Check sheet for the modelled part. Datum: model origin and axes. Units: mm. Coordinates: 2 decimals unless noted, no trailing zeros. Write each loop counter-clockwise with the first axis right and the second up, starting at its lowest first coordinate (ties: lowest second). Pieces come first, ordered by that corner, then holes. Notation, with made-up numbers: (54, -30.75) - (73, -30.75) arc R21 cw to (73, -8.75) - close; hole circle Ø8 at (71.25, 31.5). An arc over 180 degrees is marked (long way). Use one line per item in the form item = value. Start each with the question number.
1. Cross-section at A-A on z = -156.5. Record the boundary of the cut face in (x, y), then the cut area to 3 significant figures.
2. Go/stop test with flat-tipped pins: pin 1 Ø6 at (x, z) = (0, 195) entering from +Y; pin 2 Ø1.5 at (x, y) = (10, 1) entering from -Z; pin 3 Ø1.5 at (y, z) = (-1, -207) entering from +X. Record where each tip stops, or that it passes through.
3. Cross-section at B-B on y = 0.55. Record the boundary of the cut face in (x, z) (3 decimals).
4. Scan lines: line 1 along Z through (x, y) = (0, -0.4) (3 decimals); line 2 along X through (y, z) = (-1.35, 195) (3 decimals); line 3 along Z through (x, y) = (-4.5, -2). Record each from-to range of solid material in increasing order.
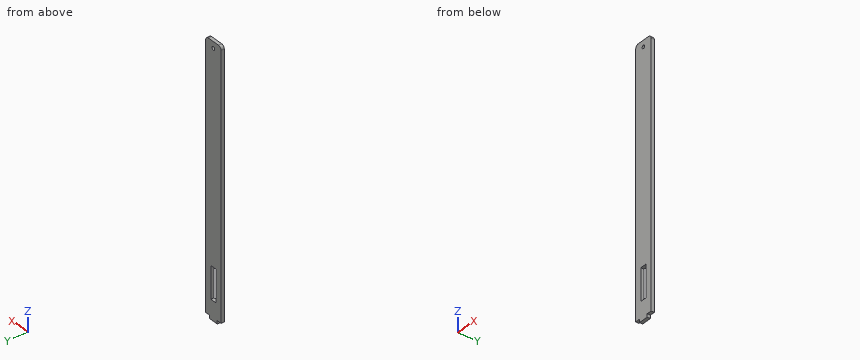
```python
from build123d import *

# Parameters (mm, degrees)
F0_W     = 15
F0_H     = 5
F1_DEPTH = 2.5
F3_D     = 5.25
F4_R     = 5
F5_W     = 10
F5_H     = 50
F6_DEPTH = 10


with BuildPart() as f1:
    # F0 (on Front) → F1 (new body, symmetric)
    with BuildSketch(Plane.XZ):
        Polygon((15, -205), (15, 205), (-15, 205), (-15, -205), (-7.5, -205), (-7.5, -200), (7.5, -200), (7.5, -205), align=None)
        with Locations((0, -207.5)):
            Rectangle(F0_W, F0_H)
        with Locations((0, -202.5)):
            Rectangle(F0_W, F0_H)
    extrude(amount=F1_DEPTH, both=True)

    # F3 (through all)
    with Locations(Plane.XZ.offset(2.5)):
        with Locations((0, 195)):
            Hole(F3_D / 2)

    # F4
    f4_edges = [f1.edges().sort_by_distance(p)[0] for p in [
        (15, 0, 205),
        (-15, 0, 205),
    ]]
    fillet(f4_edges, radius=F4_R)

    # F5 (on face) → F6 (cut)
    with BuildSketch(Plane.XZ.offset(2.5)):
        with Locations((0, -155)):
            Rectangle(F5_W, F5_H)
    extrude(amount=-F6_DEPTH, mode=Mode.SUBTRACT)


solid = f1.part
```
Final values:
q1.outline = (-15, -2.5) - (-5, -2.5) - (-5, 2.5) - (-15, 2.5) - close; (5, -2.5) - (15, -2.5) - (15, 2.5) - (5, 2.5) - close
q1.area = 100 mm²
q2.pin_1 = 2.5
q2.pin_2 = -205
q2.pin_3 = 7.5
q3.outline = (-15, -205) - (-7.5, -205) - (-7.5, -210) - (7.5, -210) - (7.5, -205) - (15, -205) - (15, 200) arc R5 ccw to (10, 205) - (-10, 205) arc R5 ccw to (-15, 200) - close; hole (-5, -180) - (5, -180) - (5, -130) - (-5, -130) - close; hole circle Ø5.25 at (0, 195)
q4.line_1 = -210 to -180, -130 to 192.375, 197.625 to 205
q4.line_2 = -15 to -2.625, 2.625 to 15
q4.line_3 = -210 to -180, -130 to 205
